For this review, take the finished solid that the model builds, in its own axes (mm). Face numbers are marked on the shaded views. A direction names the side the tool comes from. Give positions to 0.01 mm unless a question says otherwise; leave off trailing zeros. Write each loop counter-clockwise with the first axis right and the second up, starting at its lowest first coordinate (ties: lowest second). Pieces come first, ordered by that corner, then holes.
1) For P1, Ø3, axis at x = 21, z = 19.5, coming from the +Y side; P2, Ø10, axis at x = -5, z = -5.5, coming from the -Y side; P3, Ø1, axis at x = 11, z = -3, coming from the +Y side, all flat-tipped, find the tip position at first contact; note any pin that passes through.
2) We need section C-C on y = 8. Give the boundary of the cut face in (x, z), and give its area (3 significant figures).
3) We need section B-B on z = 11. Give the boundary of the cut face in (x, y), and give its area (3 significant figures).
4) We need section D-D on x = -9.5. Give the boundary of the cut face in (y, z), and give its area (3 significant figures).
5) Draft analysis for pull direction X (two halves, no side actions). For the marked faces 3, 4 and 5, state which applies: pulls with the +X half, pulls with the -X half, needs draft (parallel to the pull), parting line crosses it, or undercut.
6) Machinability: for the marked faces 1 and 2, which of the approach directions +Z, -Z, +X, -X, +Y, -Y give a long, thin tool a straight path to every point of the face, cutting with its end or side? Answer none if there is none.
7) Wall thickness on line 1 along X through (y, z) = (0.8, 20); line 2 along Z through (x, y) = (-20, 1); line 3 along Z through (x, y) = (-20, 3): over which ranges is each line inside the solid? List them lowest first.
8) We need section A-A on x = 20. Give the boundary of the cut face in (y, z).
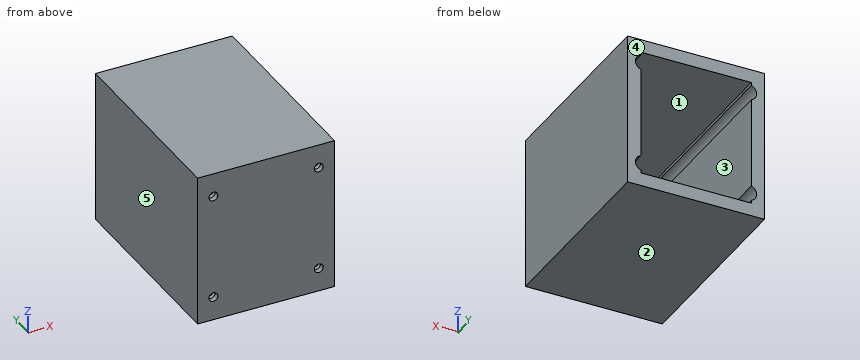
from build123d import *

# Parameters (mm, degrees)
SKETCH1_W           = 52
SKETCH1_H           = 58
SKETCH1_R           = 1.7
BOSS_EXTRUDE1_DEPTH = 2
SKETCH2_W           = 52
SKETCH2_H           = 58
SKETCH2_R           = 3
BOSS_EXTRUDE2_DEPTH = 3
SKETCH3_W           = 52
SKETCH3_H           = 58
BOSS_EXTRUDE3_DEPTH = 70


with BuildPart() as part:
    # Sketch1 → Boss-Extrude1 (new body)
    with BuildSketch(Plane(origin=(0, 0, 0), x_dir=(1, 0, 0), z_dir=(0, 1, 0))):
        Rectangle(SKETCH1_W, SKETCH1_H)
        with Locations((-20, 20)):
            Circle(SKETCH1_R, mode=Mode.SUBTRACT)
        with Locations((-20, -20)):
            Circle(SKETCH1_R, mode=Mode.SUBTRACT)
        with Locations((20, -20)):
            Circle(SKETCH1_R, mode=Mode.SUBTRACT)
        with Locations((20, 20)):
            Circle(SKETCH1_R, mode=Mode.SUBTRACT)
    extrude(amount=BOSS_EXTRUDE1_DEPTH)

    # Sketch2 → Boss-Extrude2 (add)
    with BuildSketch(Plane(origin=(0, 2, 0), x_dir=(1, 0, 0), z_dir=(0, 1, 0))):
        Rectangle(SKETCH2_W, SKETCH2_H)
        with Locations((-20, 20)):
            Circle(SKETCH2_R, mode=Mode.SUBTRACT)
        with Locations((-20, -20)):
            Circle(SKETCH2_R, mode=Mode.SUBTRACT)
        with Locations((20, 20)):
            Circle(SKETCH2_R, mode=Mode.SUBTRACT)
        with Locations((20, -20)):
            Circle(SKETCH2_R, mode=Mode.SUBTRACT)
    extrude(amount=BOSS_EXTRUDE2_DEPTH)

    # Sketch3 → Boss-Extrude3 (add)
    with BuildSketch(Plane(origin=(0, 5, 0), x_dir=(1, 0, 0), z_dir=(0, 1, 0))):
        Rectangle(SKETCH3_W, SKETCH3_H)
        with BuildLine():
            Line((-21, 22.828427125), (-21, 24))
            Line((-21, 24), (21, 24))
            Line((21, 24), (21, 22.828427125))
            ThreePointArc((21, 22.828427125), (22.449489743, 21.732050808), (23, 20))
            ThreePointArc((23, 20), (22.449489743, 18.267949192), (21, 17.171572875))
            Line((21, 17.171572875), (21, -17.171572875))
            ThreePointArc((21, -17.171572875), (22.449489743, -18.267949192), (23, -20))
            ThreePointArc((23, -20), (22.449489743, -21.732050808), (21, -22.828427125))
            Line((21, -22.828427125), (21, -24))
            Line((21, -24), (-21, -24))
            Line((-21, -24), (-21, -22.828427125))
            ThreePointArc((-21, -22.828427125), (-23, -20), (-21, -17.171572875))
            Line((-21, -17.171572875), (-21, 17.171572875))
            ThreePointArc((-21, 17.171572875), (-23, 20), (-21, 22.828427125))
        make_face(mode=Mode.SUBTRACT)
    extrude(amount=BOSS_EXTRUDE3_DEPTH)


solid = part.part
Results list:
1. P1: stops at y = 2
1. P2: stops at y = 0
1. P3: stops at y = 5
2. outline: (-26, -29) - (26, -29) - (26, 29) - (-26, 29) - close; hole (-21, -24) - (21, -24) - (21, -22.83) arc R3 ccw to (21, -17.17) - (21, 17.17) arc R3 ccw to (21, 22.83) - (21, 24) - (-21, 24) - (-21, 22.83) arc R3 ccw to (-21, 17.17) - (-21, -17.17) arc R3 ccw to (-21, -22.83) - close
2. area: 967 mm2
3. outline: (-26, 0) - (26, 0) - (26, 75) - (21, 75) - (21, 5) - (-21, 5) - (-21, 75) - (-26, 75) - close
3. area: 960 mm2
4. outline: (0, -29) - (75, -29) - (75, -24) - (5, -24) - (5, 24) - (75, 24) - (75, 29) - (0, 29) - close
4. area: 990 mm2
5. face 3: undercut
5. face 4: needs draft
5. face 5: pulls with the -X half
6. face 1: +Y
6. face 2: -Z, +X, -X, +Y, -Y
7. line 1: x = -26 to -21.7, -18.3 to 18.3, 21.7 to 26
7. line 2: z = -29 to -21.7, -18.3 to 18.3, 21.7 to 29
7. line 3: z = -29 to -23, -17 to 17, 23 to 29
8. outline: (0, -29) - (75, -29) - (75, -24) - (5, -24) - (5, -23) - (2, -23) - (2, -21.7) - (0, -21.7) - close; (0, -18.3) - (2, -18.3) - (2, -17) - (5, -17) - (5, 17) - (2, 17) - (2, 18.3) - (0, 18.3) - close; (0, 21.7) - (2, 21.7) - (2, 23) - (5, 23) - (5, 24) - (75, 24) - (75, 29) - (0, 29) - close
